Verification items for the finished model (mm, model axes). Face numbers are marked on the shaded views. Coordinates: 2 decimals unless noted, no trailing zeros. Write each loop counter-clockwise with the first axis right and the second up, starting at its lowest first coordinate (ties: lowest second). Pieces come first, ordered by that corner, then holes. Notation, with made-up numbers: (17, 76.25) -> (76, 76.25) arc R13 cw to (76, 80.25) -> close; hole circle Ø1 at (-32, 83.5). An arc over 180 degrees is marked (long way). Answer in a Markdown table with one row per item.
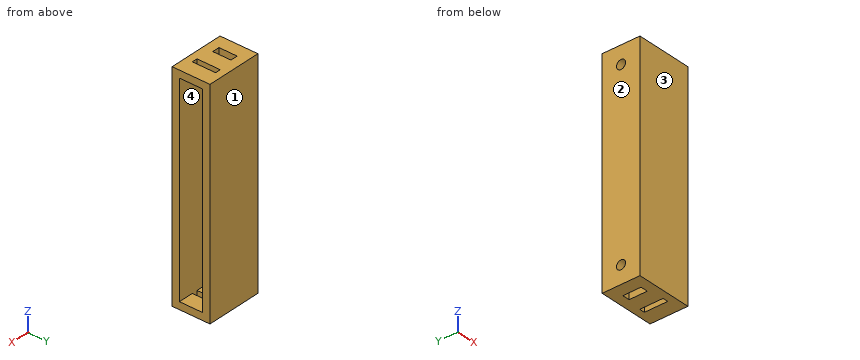
```python
from build123d import *

# Parameters (mm, degrees)
SKETCH2_W               = 111.6
SKETCH2_H               = 12.8
ARM_DEPTH               = 13.4
SHELL_T                 = 4
PIVOT_PEG_HOLE_REACH    = 122.807
SKETCH3_R               = 2.5
CABLE_PASSTHROUGH_REACH = 124.021
SKETCH4_W               = 3
SKETCH4_H               = 12.8
SKETCH4_W_2             = 4
SKETCH4_H_2             = 10


with BuildPart() as part:
    # Sketch2 → arm (new, symmetric)
    with BuildSketch(Plane(origin=(0, 0, 0), x_dir=(0, 0, -1), z_dir=(1, 0, 0))):
        with Locations((55.8, 6.4)):
            Rectangle(SKETCH2_W, SKETCH2_H)
    extrude(amount=ARM_DEPTH, both=True)

    # shell
    shell_openings = [part.faces().sort_by_distance(p)[0] for p in [
        (13.4, 6.4, -55.8),
    ]]
    offset(amount=SHELL_T, openings=shell_openings, kind=Kind.INTERSECTION)

    # Sketch3 → pivot peg hole (cut, up to next)
    with BuildSketch(Plane.ZY.offset(17.4), mode=Mode.PRIVATE) as pivot_peg_hole_sk1:
        with Locations((-5.8, 6.4)):
            Circle(SKETCH3_R)
    pivot_peg_hole_tool1 = extrude(pivot_peg_hole_sk1.sketch, amount=-PIVOT_PEG_HOLE_REACH, mode=Mode.PRIVATE) & part.part
    pivot_peg_hole = pivot_peg_hole_tool1.solids().sort_by_distance((-17.4, 6.4, -5.8))[0]
    add(pivot_peg_hole, mode=Mode.SUBTRACT)

    # Sketch4 → cable passthrough (cut, up to next)
    with BuildSketch(Plane.XY.offset(4), mode=Mode.PRIVATE) as cable_passthrough_sk1:
        with Locations((3.6, 6.4)):
            Rectangle(SKETCH4_W, SKETCH4_H)
    cable_passthrough_tool1 = extrude(cable_passthrough_sk1.sketch, amount=-CABLE_PASSTHROUGH_REACH, mode=Mode.PRIVATE) & part.part
    # Sketch4 → cable passthrough (cut, up to next)
    with BuildSketch(Plane.XY.offset(4), mode=Mode.PRIVATE) as cable_passthrough_sk2:
        with Locations((-8.4, 6.4)):
            Rectangle(SKETCH4_W_2, SKETCH4_H_2)
    cable_passthrough_tool2 = extrude(cable_passthrough_sk2.sketch, amount=-CABLE_PASSTHROUGH_REACH, mode=Mode.PRIVATE) & part.part
    cable_passthrough_1 = cable_passthrough_tool1.solids().sort_by_distance((3.6, 6.4, 4))[0]
    add(cable_passthrough_1, mode=Mode.SUBTRACT)
    cable_passthrough_2 = cable_passthrough_tool2.solids().sort_by_distance((-8.4, 6.4, 4))[0]
    add(cable_passthrough_2, mode=Mode.SUBTRACT)
    cable_passthrough = cable_passthrough_1 + cable_passthrough_2  # cable passthrough as one shape, for the pattern or mirror that repeats it

    # elbow mount: pivot peg hole, cable passthrough across plane
    add(pivot_peg_hole.mirror(Plane.XY.offset(-55.8)), mode=Mode.SUBTRACT)
    add(cable_passthrough.mirror(Plane.XY.offset(-55.8)), mode=Mode.SUBTRACT)


solid = part.part
```
1. Go/stop test with a flat-tipped pin: pin 1 (12 mm diameter, centred on y = 4.5, z = -10.5, fed in from +X). Record where the tip stops, or that it passes through.
Findings below:
| item | result |
|---|---|
| pin 1 | stops at x = 13.4 |
2. Sectioned sample at C-C, the plane y = 6.4. Count the separate pieces of the cut face and the enclosed holes in it, and give its area (3 significant figures).
Findings below:
| item | result |
|---|---|
| separate pieces | 7 |
| enclosed holes | 0 |
| area | 597 mm² |
3. Sectioned sample at A-A, the plane z = -105.8. Record the cut outline in (x, y), and give its area (3 significant figures).
Findings below:
| item | result |
|---|---|
| outline | (-17.4, -4) -> (13.4, -4) -> (13.4, 0) -> (-13.4, 0) -> (-13.4, 3.9) -> (-17.4, 3.9) -> close; (-17.4, 8.9) -> (-13.4, 8.9) -> (-13.4, 12.8) -> (13.4, 12.8) -> (13.4, 16.8) -> (-17.4, 16.8) -> close |
| area | 278 mm² |
4. Sectioned sample at B-B, the plane x = -4.5. Record the cut outline in (y, z), and give its area (3 significant figures).
Findings below:
| item | result |
|---|---|
| outline | (-4, -115.6) -> (16.8, -115.6) -> (16.8, 4) -> (-4, 4) -> close; hole (0, -111.6) -> (12.8, -111.6) -> (12.8, 0) -> (0, 0) -> close |
| area | 1,060 mm² |
5. Material ranges on probe 1 along Y at (x, z) = (9, -91); probe 2 along Z at (x, y) = (-13, 0.75); probe 3 along Y at (x, z) = (-15.25, -5.8), recorded low to high. Write a range as from..to.
Findings below:
| item | result |
|---|---|
| probe 1 | y = -4..0, 12.8..16.8 |
| probe 2 | z = -115.6..-111.6, 0..4 |
| probe 3 | y = -4..3.9, 8.9..16.8 |
6. Sectioned sample at D-D, the plane z = -58.5. Record the cut outline in (x, y).
Findings below:
| item | result |
|---|---|
| outline | (-17.4, -4) -> (13.4, -4) -> (13.4, 0) -> (-13.4, 0) -> (-13.4, 12.8) -> (13.4, 12.8) -> (13.4, 16.8) -> (-17.4, 16.8) -> close |
7. Release check for a two-part mould opening along Y. For the marked faces 1, 2, 3 and 4 record: released by +Y, released by -Y, zero draft, split by the parting line, or undercut.
Findings below:
| item | result |
|---|---|
| face 1 | released by +Y |
| face 2 | zero draft |
| face 3 | released by -Y |
| face 4 | undercut |
